```python
from build123d import *

# Parameters (mm, degrees)
SKETCH_W     = 75
SKETCH_H     = 30
SKETCH_R     = 1.75
SKETCH_W_2   = 15
SKETCH_H_2   = 20
PAD_DEPTH    = 5
FILLET_R     = 10
FILLET001_R  = 1
SKETCH001_W  = 5
SKETCH001_H  = 30
PAD001_DEPTH = 30
FILLET002_R  = 5
FILLET003_R  = 5
SKETCH002_R  = 2.75
POCKET_DEPTH = 75.001
CHAMFER_SIZE = 10


with BuildPart() as part:
    # Sketch → Pad (new body)
    with BuildSketch(Plane.XY):
        with Locations((27.5, 0)):
            Rectangle(SKETCH_W, SKETCH_H)
        Circle(SKETCH_R, mode=Mode.SUBTRACT)
        with Locations((40, 0)):
            Circle(SKETCH_R, mode=Mode.SUBTRACT)
        with Locations((20, 0)):
            Rectangle(SKETCH_W_2, SKETCH_H_2, mode=Mode.SUBTRACT)
    extrude(amount=PAD_DEPTH)

    # Fillet
    fillet_edges = [part.edges().sort_by_distance(p)[0] for p in [
        (-10, 15, 2.5),
        (-10, -15, 2.5),
    ]]
    fillet(fillet_edges, radius=FILLET_R)

    # Fillet001
    fillet001_edges = [part.edges().sort_by_distance(p)[0] for p in [
        (12.5, 0, 5),
        (12.5, 0, 0),
        (20, 10, 0),
        (20, 10, 5),
        (27.5, 0, 5),
        (20, -10, 5),
        (27.5, 0, 0),
        (20, -10, 0),
    ]]
    fillet(fillet001_edges, radius=FILLET001_R)

    # Sketch001 (on Face18 of Fillet001) → Pad001 (join)
    with BuildSketch(Plane.XY.offset(5)):
        with Locations((62.5, 0)):
            Rectangle(SKETCH001_W, SKETCH001_H)
    extrude(amount=PAD001_DEPTH)

    # Fillet002
    fillet002_edges = [part.edges().sort_by_distance(p)[0] for p in [
        (65, 0, 0),
    ]]
    fillet(fillet002_edges, radius=FILLET002_R)

    # Fillet003
    fillet003_edges = [part.edges().sort_by_distance(p)[0] for p in [
        (60, 0, 5),
    ]]
    fillet(fillet003_edges, radius=FILLET003_R)

    # Sketch002 (on Face9 of Fillet003) → Pocket (cut, through all)
    with BuildSketch(Plane.YZ.offset(65)):
        with Locations((0, 29)):
            Circle(SKETCH002_R)
        with Locations((0, 14)):
            Circle(SKETCH002_R)
    extrude(amount=-POCKET_DEPTH, mode=Mode.SUBTRACT)

    # Chamfer
    chamfer_edges = [part.edges().sort_by_distance(p)[0] for p in [
        (62.5, -15, 35),
        (62.5, 15, 35),
    ]]
    chamfer(chamfer_edges, length=CHAMFER_SIZE)


solid = part.part
```
Geometry: final body of the model. Coordinates: model frame, mm. A direction names the side the tool comes from. Round coordinates to 2 decimals unless told otherwise and drop trailing zeros. Order: outer loops, then holes, each group sorted by start corner. A loop starts at its lowest first (then second) coordinate and runs counter-clockwise, first axis right, second up. Notation, with made-up numbers: M 87,-23.5 L 103,-23.5 A16 cw 103,-0.5 Z; hole C -18.5,19 d7. An arc over 180 degrees is marked long. One line per item, written item: value.
(1) Cut plane A-A (x = 20). Return the cut outline in (y, z).
Result sheet:
outline: M -15,0 L -11,0 A1 ccw -10,1 L -10,4 A1 ccw -11,5 L -15,5 Z; M 10,1 A1 ccw 11,0 L 15,0 L 15,5 L 11,5 A1 ccw 10,4 Z
(2) Cut plane D-D (x = 40). Return the cut outline in (y, z).
Result sheet:
outline: M -15,0 L -1.75,0 L -1.75,5 L -15,5 Z; M 1.75,0 L 15,0 L 15,5 L 1.75,5 Z
(3) Cut plane C-C (y = 1). Give the number of separate pieces and of enclosed holes in the cut face, and give its area (3 significant figures).
Result sheet:
separate pieces: 6
enclosed holes: 0
area: 369 mm2
(4) Pin query (flat end, axial travel): P1, Ø4, axis at y = 7.5, z = 25.5, coming from the -X side; P2, Ø4.5, axis at x = 40, y = 0, coming from the +Z side; P3, Ø2.5, axis at y = -0.5, z = 3, coming from the +X side. Return the tip coordinate at first contact, or that it passes through.
Result sheet:
P1: x = 60
P2: z = 5
P3: x = 64.94
(5) Pull-direction query (Y, two-part tool) for faces 4 (the flat face through (65, 0, 20)), 5 (the flat face through (27.5, 0, 2)), 6 (the cylindrical face through (-7.15, -11.99, 2.54)); classes: pulls with the +Y half, pulls with the -Y half, needs draft (parallel to the pull), parting line crosses it, or undercut.
Result sheet:
face 4: needs draft
face 5: undercut
face 6: pulls with the -Y half
(6) Line query: probe 1 along Y at (x, z) = (40, 3.5); probe 2 along Z at (x, y) = (61.45, 0); probe 3 along Z at (x, y) = (62, 0). Output: solid intervals per line, ascending. Write a range as [from, to].
Result sheet:
probe 1: [-15, -1.75], [1.75, 15]
probe 2: [0.21, 11.25], [16.75, 26.25], [31.75, 35]
probe 3: [0.42, 11.25], [16.75, 26.25], [31.75, 35]
(7) Reachability of faces 1 (the flat face through (62, 0, 35)), 2 (the flat face through (29, 0, 5)), 3 (the flat face through (12.5, 0, 2)) from +Z, -Z, +X, -X, +Y, -Y: full face, straight path, thin tool, end or side. Return the list, or none.
Result sheet:
face 1: +Z, +X, -X, +Y, -Y
face 2: +Z, -X, +Y, -Y
face 3: +Z, -Z
(8) Cut plane B-B (z = 14). Return the cut outline in (x, y).
Result sheet:
outline: M 60,-15 L 65,-15 L 65,-2.75 L 60,-2.75 Z; M 60,2.75 L 65,2.75 L 65,15 L 60,15 Z
